from build123d import *

# Parameters (mm, degrees)
SALIENTE_EXTRUIR2_DEPTH = 31
CORTAR_EXTRUIR1_DEPTH   = 10
REDONDEO4_R             = 15
REDONDEO7_R             = 30
SALIENTE_EXTRUIR3_DEPTH = 5
REDONDEO8_R             = 4
REDONDEO9_R             = 4
REDONDEO11_R            = 4


with BuildPart() as part:
    # Croquis2 → Saliente-Extruir2 (new body)
    with BuildSketch(Plane(origin=(0, 0, 0), x_dir=(1, 0, 0), z_dir=(0, 1, 0))):
        Polygon((-84.881784923, 58.155199905), (-84.881784923, 55.155199905), (-46.280707897, 55.155199905), (0, 0), (46.398922974, 0), (46.398922974, 3), (1.398922974, 3), (-44.881784923, 58.155199905), align=None)
    extrude(amount=SALIENTE_EXTRUIR2_DEPTH)

    # Croquis3 → Cortar-Extruir1 (cut)
    with BuildSketch(Plane(origin=(0, 0, -58.155199905), x_dir=(-1, 0, 0), z_dir=(0, 0, -1))):
        with BuildLine():
            Line((58.164270502, 25.045941546), (62.406911189, 20.803300859))
            ThreePointArc((62.406911189, 20.803300859), (62.406911189, 17.974873734), (59.578484064, 17.974873734))
            Line((59.578484064, 17.974873734), (55.335843377, 22.217514421))
            ThreePointArc((55.335843377, 22.217514421), (55.335843377, 25.045941546), (58.164270502, 25.045941546))
        make_face()
        with BuildLine():
            Line((71.599299344, 5.954058454), (67.356658657, 10.196699141))
            ThreePointArc((67.356658657, 10.196699141), (67.356658657, 13.025126266), (70.185085782, 13.025126266))
            Line((70.185085782, 13.025126266), (74.427726469, 8.782485579))
            ThreePointArc((74.427726469, 8.782485579), (74.427726469, 5.954058454), (71.599299344, 5.954058454))
        make_face()
        with BuildLine():
            Line((74.427726469, 22.217514421), (70.185085782, 17.974873734))
            ThreePointArc((70.185085782, 17.974873734), (67.356658657, 17.974873734), (67.356658657, 20.803300859))
            Line((67.356658657, 20.803300859), (71.599299344, 25.045941546))
            ThreePointArc((71.599299344, 25.045941546), (74.427726469, 25.045941546), (74.427726469, 22.217514421))
        make_face()
        with BuildLine():
            Line((55.335843377, 8.782485579), (59.578484064, 13.025126266))
            ThreePointArc((59.578484064, 13.025126266), (62.406911189, 13.025126266), (62.406911189, 10.196699141))
            Line((62.406911189, 10.196699141), (58.164270502, 5.954058454))
            ThreePointArc((58.164270502, 5.954058454), (55.335843377, 5.954058454), (55.335843377, 8.782485579))
        make_face()
    extrude(amount=-CORTAR_EXTRUIR1_DEPTH, mode=Mode.SUBTRACT)

    # Redondeo4
    redondeo4_edges = [part.edges().sort_by_distance(p)[0] for p in [
        (-84.881784923, 0, -56.655199905),
        (-84.881784923, 31, -56.655199905),
    ]]
    fillet(redondeo4_edges, radius=REDONDEO4_R)

    # Redondeo7
    # the kernel refuses this fillet: 30 mm, written as the material it takes off along each edge
    with BuildSketch(Plane(origin=(46.398922974, 0, 75), x_dir=(-1, 0, 0), z_dir=(0, 0, -1))) as redondeo7_piece_1:
        with BuildLine():
            CenterArc((REDONDEO7_R, REDONDEO7_R), REDONDEO7_R, 180, 90)
            Line((0, REDONDEO7_R), (0, 0))
            Line((0, 0), (REDONDEO7_R, 0))
        make_face()
    extrude(amount=153, mode=Mode.SUBTRACT)
    with BuildSketch(Plane(origin=(46.398922974, 31, 75), x_dir=(-1, 0, 0), z_dir=(0, 0, -1))) as redondeo7_piece_2:
        with BuildLine():
            CenterArc((REDONDEO7_R, -REDONDEO7_R), REDONDEO7_R, 90, 90)
            Line((0, -REDONDEO7_R), (0, 0))
            Line((0, 0), (REDONDEO7_R, 0))
        make_face()
    extrude(amount=153, mode=Mode.SUBTRACT)

    # Croquis4 → Saliente-Extruir3 (add, symmetric)
    with BuildSketch(Plane(origin=(0, 15.5, 0), x_dir=(1, 0, 0), z_dir=(0, 1, 0))):
        Polygon((-8.108577144, 14.330597423), (16.398922974, 3), (1.398922974, 3), align=None)
        Polygon((-52.760428047, 55.155199905), (-41.234854299, 49.141785751), (-46.280707897, 55.155199905), align=None)
    extrude(amount=SALIENTE_EXTRUIR3_DEPTH, both=True)

    # Redondeo8
    redondeo8_edges = [part.edges().sort_by_distance(p)[0] for p in [
        (4.145172915, 20.5, -8.665298711),
    ]]
    fillet(redondeo8_edges, radius=REDONDEO8_R)

    # Redondeo9
    redondeo9_edges = [part.edges().sort_by_distance(p)[0] for p in [
        (4.145172915, 10.5, -8.665298711),
    ]]
    fillet(redondeo9_edges, radius=REDONDEO9_R)

    # Redondeo11
    # the kernel refuses this fillet: 4 mm, written as the material it takes off along each edge
    with BuildSketch(Plane(origin=(-61.626254007, 10.5, -59.780903099), x_dir=(0, 1, 0), z_dir=(0.886582596003956, 0, 0.4625703194789808))) as redondeo11_piece_1_section:
        with BuildLine():
            CenterArc((REDONDEO11_R, -REDONDEO11_R), REDONDEO11_R, 90, 90)
            Line((0, -REDONDEO11_R), (0, 0))
            Line((0, 0), (REDONDEO11_R, 0))
        make_face()
    redondeo11_piece_1 = extrude(amount=33, mode=Mode.PRIVATE)
    redondeo11_piece_1 = split(redondeo11_piece_1, bisect_by=Plane(origin=(-45.320912512, 11.608841442, -54.011360305), z_dir=(-0.7660444431189792, 0, 0.642787609686538)), keep=Keep.TOP, mode=Mode.PRIVATE)
    redondeo11_piece_1 = split(redondeo11_piece_1, bisect_by=Plane(origin=(-46.861736651, 11.608841442, -55.155199905), z_dir=(0, 0, 1)), keep=Keep.TOP, mode=Mode.PRIVATE)
    add(redondeo11_piece_1, mode=Mode.SUBTRACT)
    with BuildSketch(Plane(origin=(-61.626254007, 20.5, -59.780903099), x_dir=(0.4625703194789808, 0, -0.886582596003956), z_dir=(0.886582596003956, 0, 0.4625703194789808))) as redondeo11_piece_2_section:
        with BuildLine():
            CenterArc((REDONDEO11_R, -REDONDEO11_R), REDONDEO11_R, 90, 90)
            Line((0, -REDONDEO11_R), (0, 0))
            Line((0, 0), (REDONDEO11_R, 0))
        make_face()
    redondeo11_piece_2 = extrude(amount=33, mode=Mode.PRIVATE)
    redondeo11_piece_2 = split(redondeo11_piece_2, bisect_by=Plane(origin=(-45.320912512, 19.391158558, -54.011360306), z_dir=(-0.7660444431189792, 0, 0.642787609686538)), keep=Keep.TOP, mode=Mode.PRIVATE)
    redondeo11_piece_2 = split(redondeo11_piece_2, bisect_by=Plane(origin=(-46.861736651, 19.391158558, -55.155199905), z_dir=(0, 0, 1)), keep=Keep.TOP, mode=Mode.PRIVATE)
    add(redondeo11_piece_2, mode=Mode.SUBTRACT)


solid = part.part
Model file for the job. Use its own axes, mm. A direction names the side the tool comes from. Coordinates: 2 decimals unless noted, no trailing zeros. Order: outer loops, then holes, each group sorted by start corner. A loop starts at its lowest first (then second) coordinate and runs counter-clockwise, first axis right, second up. Notation, with made-up numbers: M -13.5,-28 L 25.5,-28 A30 ccw 25.5,1 Z; hole C -30,29 d6. An arc over 180 degrees is marked long. Return JSON: item names as keys, results as strings.
1. Saw through at B-B (x = 35). Give the cut face in (y, z).
Ans:
{"outline": "M 6.46,-3 L 24.54,-3 L 24.54,0 L 6.46,0 Z"}
2. Pull direction Y, two halves, no side cores. Call faces 1 (the face through (-57.487, 20.066, -56.676)), 2 (the face through (2, 20.5, -4)), 3 (the face through (-80.604, 4.511, -56.634)): +Y half, -Y half, draft (parallel to the pull), parting line (faces both ways), or undercut.
Ans:
{"face 1": "undercut", "face 2": "+Y half", "face 3": "-Y half"}
3. Tool access for faces 4 (the face through (-57.427, 10.874, -56.676)), 5 (the face through (4.02, 12.24, -7.95)): list every direction of +Z, -Z, +X, -X, +Y, -Y with a clear straight run to the whole face (end or side of a thin tool).
Ans:
{"face 4": "+Z, -Z", "face 5": "-Z, +X, -Y"}
4. Flat gauge pins, fed straight in: pin 1 (8 mm diameter, centred on y = 11, z = -50.5, fed in from -X); pin 2 (2 mm diameter, centred on y = 26, z = -16.5, fed in from +X); pin 3 (5 mm diameter, centred on y = 26.5, z = -38, fed in from +X). Where does each tip first touch, or does it go through?
Ans:
{"pin 1": "x = -49.87", "pin 2": "x = -9.09", "pin 3": "x = -25.87"}
5. Drill centre lines: probe 1 along Z at (x, y) = (24, 12); probe 2 along Z at (x, y) = (-67, 10); probe 3 along X at (y, z) = (27, -33). Where is each one in solid material? Low to high.
Ans:
{"probe 1": "-3 to 0", "probe 2": "-58.16 to -55.16", "probe 3": "-27.69 to -23.77"}
6. Saw through at A-A (y = 27.5). Give the cut face in (x, z).
Ans:
{"outline": "M -79.51,-58.16 L -44.88,-58.16 L 1.4,-3 L 30.46,-3 L 30.46,0 L 0,0 L -46.28,-55.16 L -79.51,-55.16 Z"}
7. Saw through at C-C (z = -31). Give the cut face in (x, y).
Ans:
{"outline": "M -26.01,0 L -22.1,0 L -22.1,31 L -26.01,31 Z"}
